The listing builds one solid part. Answer for the finished solid, in the listing's coordinates (mm). A direction names the side the tool comes from. Give positions to 0.01 mm unless a question says otherwise; leave off trailing zeros. Answer in a Markdown table with one row per item.
Autodesk Inventor part; units mm, degrees
ref_plane "YZ Plane" through (0, 0, 0) normal (1, 0, 0) x (0, 1, 0)
ref_plane "XZ Plane" through (0, 0, 0) normal (0, 1, 0) x (-1, 0, 0)
ref_plane "XY Plane" through (0, 0, 0) normal (0, 0, 1) x (1, 0, 0)
sketch "스케치1" plane through (0, 0, 0) normal (0, 0, 1) x (1, 0, 0)
  circle A0 centre (7.7782, 7.7782) radius 1.25
  circle A1 centre (-7.7782, 7.7782) radius 1.25
  circle A2 centre (7.7782, -7.7782) radius 1.25
  circle A3 centre (-11, 0) radius 1.25
  circle A4 centre (11, 0) radius 1.25
  circle A5 centre (0, 11) radius 1.25
  circle A6 centre (0, -11) radius 1.25
  circle A7 centre (-7.7782, -7.7782) radius 1.25
  circle A8 centre (0, 0) radius 14
  circle A9 centre (0, 0) radius 5
  circle A10 centre (0, 0) radius 5
  line L0 (5, 0) -> (5, -10)
  line L1 (5, -10) -> (-5, -10)
  line L2 (-5, -10) -> (-5, 0)
  line L3 (15, -10) -> (-15, -10)
  line L4 (-15, -10) -> (-15, 195)
  line L5 (-15, 195) -> (15, 195)
  line L6 (15, 195) -> (15, -10)
  line L7 (0, 195) -> (0, 165)
  line L8 (0, 165) -> (4.2095, 175.1627)
  line L9 (0, 165) -> (11, 165) construction
  circle A11 centre (4.2095, 175.1627) radius 1.25
  circle A12 centre (-4.2095, 175.1627) radius 1.25
  circle A13 centre (-10.1627, 169.2095) radius 1.25
  circle A14 centre (-10.1627, 160.7905) radius 1.25
  circle A15 centre (-4.2095, 154.8373) radius 1.25
  circle A16 centre (4.2095, 154.8373) radius 1.25
  circle A17 centre (10.1627, 160.7905) radius 1.25
  circle A18 centre (10.1627, 169.2095) radius 1.25
  dimension "d0" = 10
  dimension "d2" = 30
  dimension "d3" = 205
  dimension "d4" = 30
  dimension "d6" = 11
  dimension "d7" = 67.5
  dimension "d8" = 2.5
  dimension "d11" = 360
extrude "판1" add sketch "스케치1" along normal blind 4 contours L0 A9 L2 L3 A8 | A8 L3 L4 L5 L6 | A15 | A16
fillet "모서리 라운드1" radius 2 6 edges at (15, -10, 2) (5, -10, 2) (-5, -10, 2) (-15, -10, 2) (15, 195, 2) (-15, 195, 2)
equation "\"TransitionRadius\" = BendRadius"
properties part number "bar2"
Item 1: Find section A-A on z = 2.65. Count the separate pieces of the cut face and the enclosed holes in it, then the cut area to 3 significant figures.
Answer block:
| item | result |
|---|---|
| separate pieces | 1 |
| enclosed holes | 13 |
| area | 5,940 mm² |
Item 2: Which of the six approach directions +Z, -Z, +X, -X, +Y, -Y give full straight-line access (tool end or side, diameter ignored) to faces 5 (the face through (-5, -4, 2)), 6 (the face through (0, 94, 0))?
Answer block:
| item | result |
|---|---|
| face 5 | +Z, -Z, -Y |
| face 6 | -Z, +X, -X, +Y, -Y |
Item 3: Consider line 1 (Y direction, x = -7.75, z = 3.05); line 2 (Y direction, x = -4, z = 2.8); line 3 (Y direction, x = 8.25, z = 0.2). Determine where each line is inside the solid, lowest interval first.
Answer block:
| item | result |
|---|---|
| line 1 | -10 to -9.03, -6.53 to 6.53, 9.03 to 195 |
| line 2 | 3 to 173.93, 176.4 to 195 |
| line 3 | -10 to -8.94, -6.62 to 6.62, 8.94 to 195 |
Item 4: Determine the mould class of faces 1 (the face through (0, 94, 4)), 2 (the face through (-15, 91, 2)), 3 (the face through (5, -4, 2)), 4 (the face through (15, 94, 2)) for opening direction X: pulls with the +X half, pulls with the -X half, needs draft (parallel to the pull), parting line crosses it, or undercut.
Answer block:
| item | result |
|---|---|
| face 1 | needs draft |
| face 2 | pulls with the -X half |
| face 3 | undercut |
| face 4 | pulls with the +X half |
Item 5: Each of these flat-tipped pins is pushed along its axis until it touches: P1, Ø1.5, axis at x = 0.5, y = 17, coming from the -Z side; P2, Ø2, axis at x = -10.16, y = 169.21, coming from the -Z side. Where does it stop, or does it pass through?
Answer block:
| item | result |
|---|---|
| P1 | z = 0 |
| P2 | through |
